from build123d import *

# Parameters (mm, degrees)
F1_DEPTH  = 2
F2_DEPTH  = 6
F3_R      = 2.5
F4_DEPTH  = 1.5
F5_R      = 1.3
F6_DEPTH  = 1.5
F8_DEPTH  = 7
F9_R      = 1.5
F10_DEPTH = 10
F11_W     = 12.6
F11_H     = 2
F11_W_2   = 9.5
F12_DEPTH = 3.8
F13_R     = 3
F14_DEPTH = 0.4
F15_SIZE  = 1.49999
F16_W     = 19.2
F16_H     = 1.1
F17_DEPTH = 1


# Not quite as in the source:
# - a fillet or chamfer is up to 0.001 mm smaller than in the source, because OpenCascade refuses the exact size


with BuildPart() as f1:
    # F0 (on Top) → F1 (new body)
    with BuildSketch(Plane.XY):
        with BuildLine():
            Line((27.5, 38.5), (-27.5, 38.5))
            ThreePointArc((-27.5, 38.5), (-33.8639610307, 35.8639610307), (-36.5, 29.5))
            Line((-36.5, 29.5), (-36.5, 27.5))
            Line((-36.5, 27.5), (-36.5, 12.5))
            Line((-36.5, 12.5), (-36.5, -12.5))
            Line((-36.5, -12.5), (-36.5, -27.5))
            ThreePointArc((-36.5, -27.5), (-33.8639610307, -33.8639610307), (-27.5, -36.5))
            Line((-27.5, -36.5), (27.5, -36.5))
            ThreePointArc((27.5, -36.5), (33.8639610307, -33.8639610307), (36.5, -27.5))
            Line((36.5, -27.5), (36.5, -12.5))
            Line((36.5, -12.5), (36.5, 12.5))
            Line((36.5, 12.5), (36.5, 27.5))
            Line((36.5, 27.5), (36.5, 29.5))
            ThreePointArc((36.5, 29.5), (33.8639610307, 35.8639610307), (27.5, 38.5))
        make_face()
    extrude(amount=F1_DEPTH)

    # F0 (on Top) → F2 (join)
    with BuildSketch(Plane.XY):
        with BuildLine():
            Line((-36.5, 12.5), (-36.5, 27.5))
            Line((-36.5, 27.5), (-40.9, 27.5))
            ThreePointArc((-40.9, 27.5), (-43.7284271247, 26.3284271247), (-44.9, 23.5))
            Line((-44.9, 23.5), (-44.9, 16.5))
            ThreePointArc((-44.9, 16.5), (-43.7284271247, 13.6715728753), (-40.9, 12.5))
            Line((-40.9, 12.5), (-36.5, 12.5))
        make_face()
        with BuildLine():
            Line((-40.9, 25.0000007004), (-38.9999992996, 25.0000007004))
            Line((-38.9999992996, 25.0000007004), (-38.9999992996, 14.9999992996))
            Line((-38.9999992996, 14.9999992996), (-40.9, 14.9999992996))
            ThreePointArc((-40.9, 14.9999992996), (-41.960660667, 15.439339333), (-42.4000007004, 16.5))
            Line((-42.4000007004, 16.5), (-42.4000007004, 23.5))
            ThreePointArc((-42.4000007004, 23.5), (-41.960660667, 24.560660667), (-40.9, 25.0000007004))
        make_face(mode=Mode.SUBTRACT)
        with BuildLine():
            Line((-36.5, -27.5), (-36.5, -12.5))
            Line((-36.5, -12.5), (-40.9, -12.5))
            ThreePointArc((-40.9, -12.5), (-43.7284271247, -13.6715728753), (-44.9, -16.5))
            Line((-44.9, -16.5), (-44.9, -23.5))
            ThreePointArc((-44.9, -23.5), (-43.7284271247, -26.3284271247), (-40.9, -27.5))
            Line((-40.9, -27.5), (-36.5, -27.5))
        make_face()
        with BuildLine():
            Line((-38.9999992996, -14.9999992996), (-38.9999992996, -25.0000007004))
            Line((-38.9999992996, -25.0000007004), (-40.9, -25.0000007004))
            ThreePointArc((-40.9, -25.0000007004), (-41.960660667, -24.560660667), (-42.4000007004, -23.5))
            Line((-42.4000007004, -23.5), (-42.4000007004, -16.5))
            ThreePointArc((-42.4000007004, -16.5), (-41.960660667, -15.439339333), (-40.9, -14.9999992996))
            Line((-40.9, -14.9999992996), (-38.9999992996, -14.9999992996))
        make_face(mode=Mode.SUBTRACT)
        with BuildLine():
            Line((40.9, 27.5), (36.5, 27.5))
            Line((36.5, 27.5), (36.5, 12.5))
            Line((36.5, 12.5), (40.9, 12.5))
            ThreePointArc((40.9, 12.5), (43.7284271247, 13.6715728753), (44.9, 16.5))
            Line((44.9, 16.5), (44.9, 23.5))
            ThreePointArc((44.9, 23.5), (43.7284271247, 26.3284271247), (40.9, 27.5))
        make_face()
        with BuildLine():
            Line((40.9, 14.9999992996), (38.9999992996, 14.9999992996))
            Line((38.9999992996, 14.9999992996), (38.9999992996, 25.0000007004))
            Line((38.9999992996, 25.0000007004), (40.9, 25.0000007004))
            ThreePointArc((40.9, 25.0000007004), (41.960660667, 24.560660667), (42.4000007004, 23.5))
            Line((42.4000007004, 23.5), (42.4000007004, 16.5))
            ThreePointArc((42.4000007004, 16.5), (41.960660667, 15.439339333), (40.9, 14.9999992996))
        make_face(mode=Mode.SUBTRACT)
        with BuildLine():
            Line((40.9, -12.5), (36.5, -12.5))
            Line((36.5, -12.5), (36.5, -27.5))
            Line((36.5, -27.5), (40.9, -27.5))
            ThreePointArc((40.9, -27.5), (43.7284271247, -26.3284271247), (44.9, -23.5))
            Line((44.9, -23.5), (44.9, -16.5))
            ThreePointArc((44.9, -16.5), (43.7284271247, -13.6715728753), (40.9, -12.5))
        make_face()
        with BuildLine():
            Line((38.9999992996, -14.9999992996), (40.9, -14.9999992996))
            ThreePointArc((40.9, -14.9999992996), (41.960660667, -15.439339333), (42.4000007004, -16.5))
            Line((42.4000007004, -16.5), (42.4000007004, -23.5))
            ThreePointArc((42.4000007004, -23.5), (41.960660667, -24.560660667), (40.9, -25.0000007004))
            Line((40.9, -25.0000007004), (38.9999992996, -25.0000007004))
            Line((38.9999992996, -25.0000007004), (38.9999992996, -14.9999992996))
        make_face(mode=Mode.SUBTRACT)
    extrude(amount=F2_DEPTH)

    # F3 (on face) → F4 (join)
    with BuildSketch(Plane.XY.offset(2)):
        with Locations((-18.94, -30.6)):
            Circle(F3_R)
        with Locations((8.96, -30.6)):
            Circle(F3_R)
        with Locations((24.16, 20.2)):
            Circle(F3_R)
        with Locations((-24.24, 21.5)):
            Circle(F3_R)
    extrude(amount=F4_DEPTH)

    # F5 (on face) → F6 (join)
    with BuildSketch(Plane.XY.offset(3.5)):
        with Locations((-19.24, -30.6)):
            Circle(F5_R)
        with Locations((8.96, -30.6)):
            Circle(F5_R)
        with Locations((24.16, 20.2)):
            Circle(F5_R)
        with Locations((-24.24, 21.5)):
            Circle(F5_R)
    extrude(amount=F6_DEPTH)

    # F7 (on face) → F8 (join)
    with BuildSketch(Plane.XY.offset(2)):
        with BuildLine():
            Line((27.5, 38.5), (-27.5, 38.5))
            ThreePointArc((-27.5, 38.5), (-33.8639610307, 35.8639610307), (-36.5, 29.5))
            Line((-36.5, 29.5), (-36.5, -27.5))
            ThreePointArc((-36.5, -27.5), (-33.8639610307, -33.8639610307), (-27.5, -36.5))
            Line((-27.5, -36.5), (27.5, -36.5))
            ThreePointArc((27.5, -36.5), (33.8639610307, -33.8639610307), (36.5, -27.5))
            Line((36.5, -27.5), (36.5, 29.5))
            ThreePointArc((36.5, 29.5), (33.8639610307, 35.8639610307), (27.5, 38.5))
        make_face()
        Polygon((-27.5, 29.5), (-27.5, 36.5), (27.5, 36.5), (27.5, 29.5), (34.5, 29.5), (34.5, -27.5), (27.5, -27.5), (27.5, -34.5), (-27.5, -34.5), (-27.5, -27.5), (-34.5, -27.5), (-34.5, 29.5), align=None, mode=Mode.SUBTRACT)
    extrude(amount=F8_DEPTH)

    # F9 (on face) → F10 (cut)
    with BuildSketch(Plane.XY.offset(9)):
        with Locations((-31, 33)):
            Circle(F9_R)
        with Locations((31, 33)):
            Circle(F9_R)
        with Locations((-31, -31)):
            Circle(F9_R)
        with Locations((31, -31)):
            Circle(F9_R)
    extrude(amount=-F10_DEPTH, mode=Mode.SUBTRACT)

    # F11 (on face) → F12 (cut)
    with BuildSketch(Plane.XY.offset(9)):
        with Locations((11.36, 37.5)):
            Rectangle(F11_W, F11_H)
        with Locations((-18.89, 37.5)):
            Rectangle(F11_W_2, F11_H)
    extrude(amount=-F12_DEPTH, mode=Mode.SUBTRACT)

    # F13 (on face) → F14 (cut)
    with BuildSketch(Plane(origin=(0, 0, 0), x_dir=(1, 0, 0), z_dir=(0, 0, -1))):
        with Locations((31, -33)):
            Circle(F13_R)
        with Locations((-31, -33)):
            Circle(F13_R)
        with Locations((-31, 31)):
            Circle(F13_R)
        with Locations((31, 31)):
            Circle(F13_R)
    extrude(amount=-F14_DEPTH, mode=Mode.SUBTRACT)

    # F15 (size 1.5 in the source; OpenCascade refuses exactly that, so slightly less here)
    f15_edges = [f1.edges().sort_by_distance(p)[0] for p in [
        (29.5, 33, 0.4),
        (-32.5, 33, 0.4),
        (29.5, -31, 0.4),
        (-32.5, -31, 0.4),
    ]]
    chamfer(f15_edges, length=F15_SIZE)

    # F16 (on face) → F17 (cut)
    with BuildSketch(Plane.XY.offset(9)):
        with BuildLine():
            Line((-23.64, 38.5), (-27.5, 38.5))
            ThreePointArc((-27.5, 38.5), (-33.8639610307, 35.8639610307), (-36.5, 29.5))
            Line((-36.5, 29.5), (-36.5, -27.5))
            ThreePointArc((-36.5, -27.5), (-33.8639610307, -33.8639610307), (-27.5, -36.5))
            Line((-27.5, -36.5), (27.5, -36.5))
            ThreePointArc((27.5, -36.5), (33.8639610307, -33.8639610307), (36.5, -27.5))
            Line((36.5, -27.5), (36.5, 29.5))
            ThreePointArc((36.5, 29.5), (33.8639610307, 35.8639610307), (27.5, 38.5))
            Line((27.5, 38.5), (17.66, 38.5))
            Line((17.66, 38.5), (17.66, 37.4))
            Line((17.66, 37.4), (27.5, 37.4))
            ThreePointArc((27.5, 37.4), (33.0861435714, 35.0861435714), (35.4, 29.5))
            Line((35.4, 29.5), (35.4, -27.5))
            ThreePointArc((35.4, -27.5), (33.0861435714, -33.0861435714), (27.5, -35.4))
            Line((27.5, -35.4), (-27.5, -35.4))
            ThreePointArc((-27.5, -35.4), (-33.0861435714, -33.0861435714), (-35.4, -27.5))
            Line((-35.4, -27.5), (-35.4, 29.5))
            ThreePointArc((-35.4, 29.5), (-33.0861435714, 35.0861435714), (-27.5, 37.4))
            Line((-27.5, 37.4), (-23.64, 37.4))
            Line((-23.64, 37.4), (-23.64, 38.5))
        make_face()
        with Locations((-4.54, 37.95)):
            Rectangle(F16_W, F16_H)
    extrude(amount=-F17_DEPTH, mode=Mode.SUBTRACT)


solid = f1.part
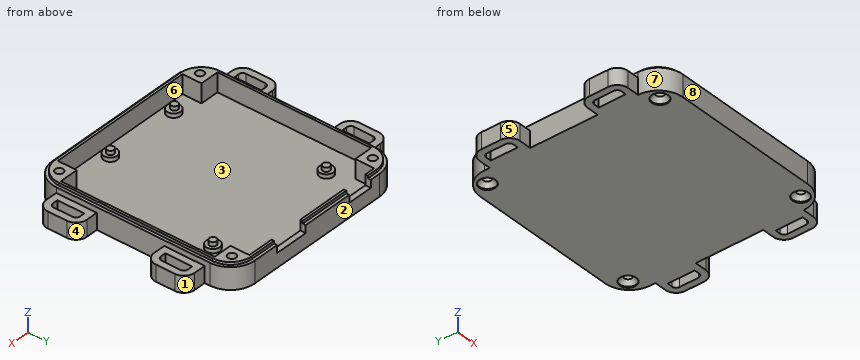
Design review of the part built by this model. Coordinates are the model's own, in mm. Face numbers are marked on the shaded views. A direction names the side the tool comes from. Round coordinates to 2 decimals unless told otherwise and drop trailing zeros. Write each loop counter-clockwise with the first axis right and the second up, starting at its lowest first coordinate (ties: lowest second). Pieces come first, ordered by that corner, then holes. Notation, with made-up numbers: (-27, 58.5) - (31, 58.5) arc R14 ccw to (31, 71.5) - close; hole circle Ø10 at (44.25, 61). An arc over 180 degrees is marked (long way). Return JSON: item names as keys, results as strings. Group by question number.
Item 1: The part is to be moulded in two halves that separate along X. For the marked faces 6, 7 and 8, say which applies: pulls with the +X half, pulls with the -X half, needs draft (parallel to the pull), parting line crosses it, or undercut.
Item 2: We need section D-D on x = -19.24. Write out the cut boundary in (y, z).
Item 3: Insertion check: P1, Ø5, axis at x = -32.5, y = -16, coming from the -Z side; P2, Ø2.5, axis at x = 41, y = 18, coming from the +Z side; P3, Ø1, axis at y = -10, z = 4, coming from the +X side; P4, Ø1, axis at y = 37.5, z = 7, coming from the +X side. Each pin has a flat end and moves straight along its axis. Give the tip position at first contact, or say it passes through.
Item 4: Machinability: for the marked faces 1, 2, 3, 4 and 5, which of the approach directions +Z, -Z, +X, -X, +Y, -Y give a long, thin tool a straight path to every point of the face, cutting with its end or side? Answer none if there is none.
Item 5: We need section B-B on y = 10. Write out the cut boundary in (x, z).
Item 6: We need section A-A on x = 0.5. Write out the cut boundary in (y, z), and give its area (3 significant figures).
Item 7: We need section C-C on x = -31. Give the number of separate pieces and of enclosed holes in the cut face, and give its area (3 significant figures).
Item 8: For probe 1 along Y at (x, z) = (41, 4.25); probe 2 along Y at (x, z) = (31, 5); probe 3 along Y at (x, z) = (-4.5, 6.5), list the stretches that pass through material, from the lowest coordinate up. Write a range as [from, to].
Model answer:
{
 "1": {"face 6": "undercut", "face 7": "pulls with the -X half", "face 8": "needs draft"},
 "2": {"outline": "(-36.5, 0) - (38.5, 0) - (38.5, 5.2) - (36.5, 5.2) - (36.5, 2) - (-28.12, 2) - (-28.12, 3.5) - (-29.3, 3.5) - (-29.3, 5) - (-31.9, 5) - (-31.9, 3.5) - (-33.08, 3.5) - (-33.08, 2) - (-34.5, 2) - (-34.5, 9) - (-35.4, 9) - (-35.4, 8) - (-36.5, 8) - close"},
 "3": {"P1": "stops at z = 0", "P2": "passes through", "P3": "stops at x = 36.5", "P4": "stops at x = 32.47"},
 "4": {"face 1": "+Z, -Z, +X, +Y", "face 2": "+Z, -Z, +X, -X, +Y", "face 3": "+Z", "face 4": "+Z, -Z, +X", "face 5": "+Z, -Z, -X"},
 "5": {"outline": "(-36.5, 0) - (36.5, 0) - (36.5, 8) - (35.4, 8) - (35.4, 9) - (34.5, 9) - (34.5, 2) - (-34.5, 2) - (-34.5, 9) - (-35.4, 9) - (-35.4, 8) - (-36.5, 8) - close"},
 "6": {"outline": "(-36.5, 0) - (38.5, 0) - (38.5, 8) - (37.4, 8) - (37.4, 9) - (36.5, 9) - (36.5, 2) - (-34.5, 2) - (-34.5, 9) - (-35.4, 9) - (-35.4, 8) - (-36.5, 8) - close", "area": "176 mm²"},
 "7": {"separate pieces": "3", "enclosed holes": "0", "area": "200 mm²"},
 "8": {"probe 1": "y = [-27.5, -25], [-15, -12.5], [12.5, 15], [25, 27.5]", "probe 2": "y = [-35.79, -32.5], [-29.5, -27.5], [29.5, 31.5], [34.5, 37.79]", "probe 3": "y = [-36.5, -34.5], [36.5, 38.5]"}
}
